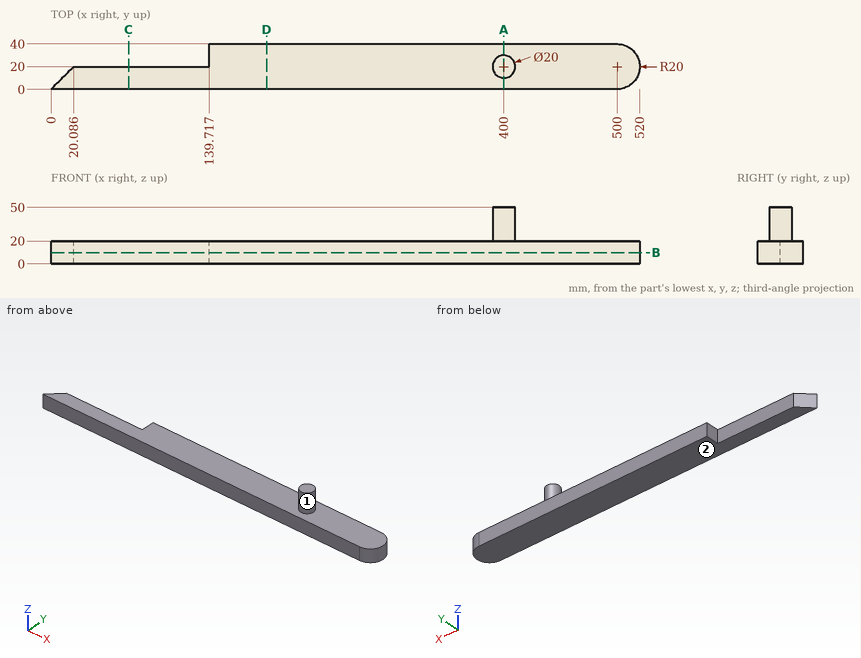
Geometry check sheet. Reference: drawing and pictorial views, mm from the part's lowest x, y, z. A direction names the side the tool comes from. Coordinates: 2 decimals unless noted, no trailing zeros. Write each loop counter-clockwise with the first axis right and the second up, starting at its lowest first coordinate (ties: lowest second). Pieces come first, ordered by that corner, then holes. Notation, with made-up numbers: M -30.5,-29.5 L -10.5,-29.5 A23 cw -10.5,1.5 Z; hole C 27.25,-26 d4. An arc over 180 degrees is marked long. Use one line per item in the form item = value.
Item 1: Sectioned sample at C-C, the plane x = 68.5. Record the cut outline in (y, z).
Answer below:
outline = M 0,0 L 20,0 L 20,20 L 0,20 Z
Item 2: Material ranges on L1, parallel to Z at x = 337.5, y = 4; L2, parallel to X at y = 12, z = 7.5; L3, parallel to X at y = 14.5, z = 17, recorded low to high. Write a range as from..to.
Answer below:
L1 = 0..20
L2 = 12.05..518.33
L3 = 14.56..519.23
Item 3: Gauge pin test, flat ends, axial feed: pin 1 Ø10 at (x, z) = (66.5, 12.5) entering from +Y; pin 2 Ø1 at (x, y) = (246.5, 8.5) entering from +Z; pin 3 Ø6 at (y, z) = (30, 13) entering from -X. Record the tip position at first contact, or that the pin passes through.
Answer below:
pin_1 = 20
pin_2 = 20
pin_3 = 139.72
Item 4: Sectioned sample at A-A, the plane x = 400. Record the cut outline in (y, z).
Answer below:
outline = M 0,0 L 40,0 L 40,20 L 30,20 L 30,50 L 10,50 L 10,20 L 0,20 Z
Item 5: Sectioned sample at D-D, the plane x = 190.5. Record the cut outline in (y, z).
Answer below:
outline = M 0,0 L 40,0 L 40,20 L 0,20 Z
Item 6: Set-up check for the marked faces 1 and 2: record each of +Z, -Z, +X, -X, +Y, -Y from which the full face is reachable in a straight line by a thin tool's end or side.
Answer below:
face_1 = +Z
face_2 = -Z, +X, -X, +Y, -Y
Item 7: Sectioned sample at B-B, the plane z = 10. Record the cut outline in (x, y), and give its area (3 significant figures).
Answer below:
outline = M 0,0 L 500,0 A20 ccw 500,40 L 139.72,40 L 139.72,20 L 20.09,20 Z
area = 17,600 mm^2
